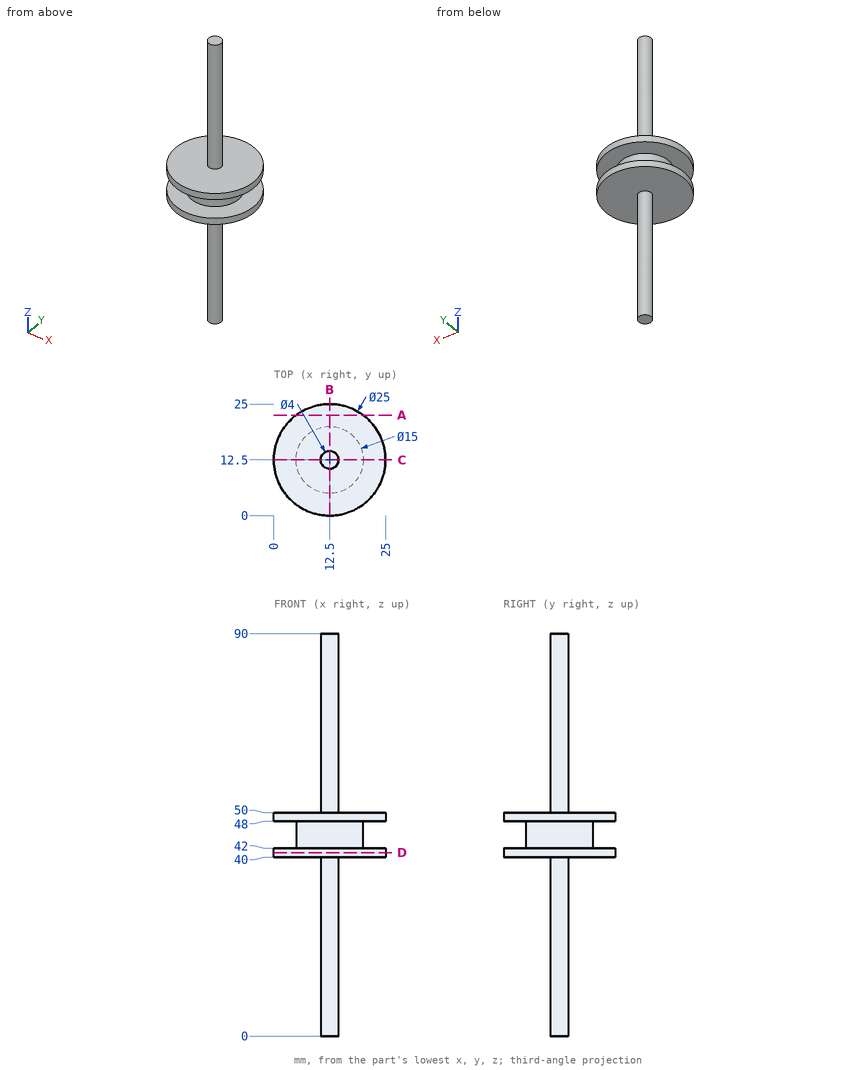
Job drawing, mm, ordinate dimensions from the low corner. One solid piece. Give positions to 0.01 mm unless a question says otherwise; leave off trailing zeros. Order: outer loops, then holes, each group sorted by start corner. A loop starts at its lowest first (then second) coordinate and runs counter-clockwise, first axis right, second up. Notation, with made-up numbers: (43.5, 4) - (76.5, 4) arc R33 ccw to (76.5, 36) - close; hole circle Ø6 at (66.5, 61.5). An arc over 180 degrees is marked (long way). Answer in a Markdown table with one row per item.
1. Saw through at D-D, the plane z = 41. Give the cut face in (x, y).
Data:
| item | result |
|---|---|
| outline | circle Ø25 at (12.5, 12.5) |
2. Saw through at A-A, the plane y = 22.5. Give the cut face in (x, z).
Data:
| item | result |
|---|---|
| outline | (5, 40) - (20, 40) - (20, 42) - (5, 42) - close; (5, 48) - (20, 48) - (20, 50) - (5, 50) - close |
3. Saw through at B-B, the plane x = 12.5. Give the cut face in (y, z).
Data:
| item | result |
|---|---|
| outline | (0, 40) - (10.5, 40) - (10.5, 0) - (14.5, 0) - (14.5, 40) - (25, 40) - (25, 42) - (20, 42) - (20, 48) - (25, 48) - (25, 50) - (14.5, 50) - (14.5, 90) - (10.5, 90) - (10.5, 50) - (0, 50) - (0, 48) - (5, 48) - (5, 42) - (0, 42) - close |
4. Flat gauge pins, fed straight in: pin 1 (2 mm diameter, centred on y = 10.5, z = 12, fed in from -X); pin 2 (6 mm diameter, centred on x = 20, y = 22, fed in from -Z); pin 3 (8 mm diameter, centred on y = 8.5, z = 55, fed in from -X). Where does each tip first touch, or does it go through?
Data:
| item | result |
|---|---|
| pin 1 | stops at x = 10.77 |
| pin 2 | stops at z = 40 |
| pin 3 | stops at x = 10.5 |
5. Probe probe 1 along Z at (x, y) = (5.25, 17); probe 2 along Z at (x, y) = (13.25, 16.5); probe 3 along X at (y, z) = (12, 68.5). List the from-to ranges inside material, lowest first. Write a range as [from, to].
Data:
| item | result |
|---|---|
| probe 1 | z = [40, 42], [48, 50] |
| probe 2 | z = [40, 50] |
| probe 3 | x = [10.56, 14.44] |
